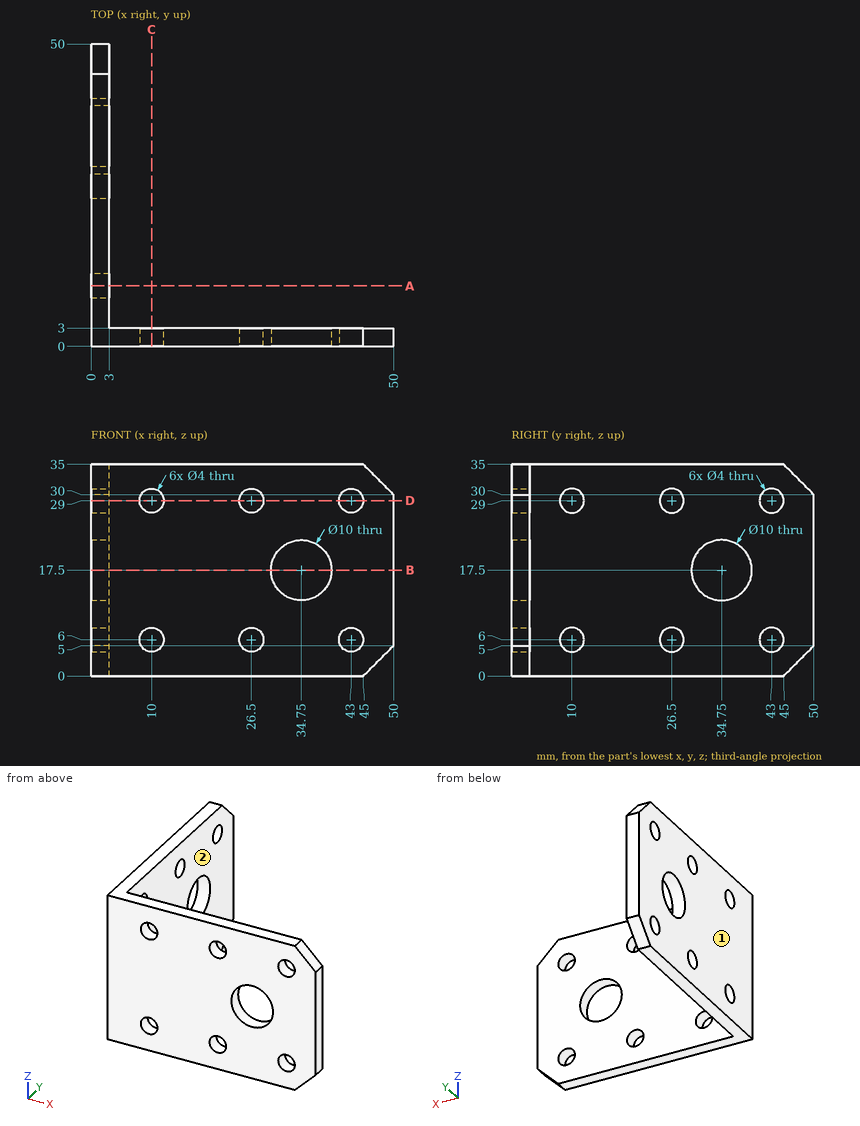
Here's the drawing with two shaded views (mm, measured from the low corner). I have some questions. A direction names the side the tool comes from. Give positions to 0.01 mm unless a question says otherwise; leave off trailing zeros. Loops run counter-clockwise (first coordinate to the right, second up) from the corner with the lowest first, then second, coordinate; pieces in that order, holes last. Notation, with made-up numbers: M 28.25,45.5 L 67.25,45.5 A7 cw 67.25,53.5 Z; hole C 24,48.25 d5. An arc over 180 degrees is marked long. One line per item, written item: value.
(1) I need wall thicknesses on line 1 (Z direction, x = 43, y = 2); line 2 (Z direction, x = 0.8, y = 34.75); line 3 (Y direction, x = 47.5, z = 19.5). Which ranges of each line are inside material? Lowest first, please.
Returned:
line 1: 0 to 4, 8 to 27, 31 to 35
line 2: 0 to 12.5, 22.5 to 35
line 3: 0 to 3
(2) Suppose I cut it at D-D on z = 29. Count the separate pieces of the cut face and the enclosed holes in it, plus the area to 3 significant figures.
Returned:
separate pieces: 7
enclosed holes: 0
area: 219 mm^2
(3) Will these pins go through, and if not, where does the flat tip stop? pin 1 (3.5 mm diameter, centred on x = 43, z = 6, fed in from -Y); pin 2 (4 mm diameter, centred on y = 27, z = 13, fed in from +X); pin 3 (4.5 mm diameter, centred on x = 43, z = 29, fed in from +Y).
Returned:
pin 1: through
pin 2: x = 3
pin 3: y = 3
(4) Suppose I cut it at A-A on y = 10. List the corners of the cut face in (x, z) for me.
Returned:
outline: M 0,0 L 3,0 L 3,4 L 0,4 Z; M 0,8 L 3,8 L 3,27 L 0,27 Z; M 0,31 L 3,31 L 3,35 L 0,35 Z
(5) Which directions (+Z, -Z, +X, -X, +Y, -Y) give clear straight access to the entire face, cutting with the end or side of a thin tool? Please do the marked faces 1 and 2.
Returned:
face 1: +Z, -Z, -X, +Y, -Y
face 2: +Z, -Z, +X, +Y
(6) Suppose I cut it at B-B on z = 17.5. List the corners of the cut face in (x, y) for me.
Returned:
outline: M 0,0 L 29.75,0 L 29.75,3 L 3,3 L 3,29.75 L 0,29.75 Z; M 0,39.75 L 3,39.75 L 3,50 L 0,50 Z; M 39.75,0 L 50,0 L 50,3 L 39.75,3 Z
